```python
from build123d import *

# Parameters (mm, degrees)
SKETCH1_R           = 12.5
BOSS_EXTRUDE1_DEPTH = 115.4
SKETCH4_W           = 8
SKETCH4_H           = 8
CUT_EXTRUDE1_DEPTH  = 35.4
SKETCH11_R          = 15.5
BOSS_EXTRUDE4_DEPTH = 2
SKETCH12_R          = 12.5
SKETCH12_R_2        = 11.75
CUT_EXTRUDE2_DEPTH  = 1.2
SKETCH13_W          = 8
SKETCH13_H          = 7
CUT_EXTRUDE3_DEPTH  = 47
SKETCH16_R          = 12.5
SKETCH16_R_2        = 11.75
CUT_EXTRUDE5_DEPTH  = 1.2


with BuildPart() as part:
    # Sketch1 → Boss-Extrude1 (new body)
    with BuildSketch(Plane.XY):
        Circle(SKETCH1_R)
    extrude(amount=BOSS_EXTRUDE1_DEPTH)

    # Sketch4 → Cut-Extrude1 (cut)
    with BuildSketch(Plane(origin=(0, 0, 0), x_dir=(-1, 0, 0), z_dir=(0, 0, -1))):
        with Locations((0, 12.5)):
            Rectangle(SKETCH4_W, SKETCH4_H)
    extrude(amount=-CUT_EXTRUDE1_DEPTH, mode=Mode.SUBTRACT)

    # Sketch11 → Boss-Extrude4 (add)
    with BuildSketch(Plane(origin=(0, 0, 37.4), x_dir=(-1, 0, 0), z_dir=(0, 0, -1))):
        Circle(SKETCH11_R)
    extrude(amount=-BOSS_EXTRUDE4_DEPTH)

    # Sketch12 → Cut-Extrude2 (cut)
    with BuildSketch(Plane.XY.offset(60)):
        Circle(SKETCH12_R)
        Circle(SKETCH12_R_2, mode=Mode.SUBTRACT)
    extrude(amount=CUT_EXTRUDE2_DEPTH, mode=Mode.SUBTRACT)

    # Sketch13 → Cut-Extrude3 (cut)
    with BuildSketch(Plane.XY.offset(115.4)):
        with Locations((0, 12.5)):
            Rectangle(SKETCH13_W, SKETCH13_H)
    extrude(amount=-CUT_EXTRUDE3_DEPTH, mode=Mode.SUBTRACT)

    # Sketch16 → Cut-Extrude5 (cut)
    with BuildSketch(Plane.XY.offset(110.4)):
        Circle(SKETCH16_R)
        Circle(SKETCH16_R_2, mode=Mode.SUBTRACT)
    extrude(amount=CUT_EXTRUDE5_DEPTH, mode=Mode.SUBTRACT)


solid = part.part
```
For this review, take the finished solid that the model builds, in its own axes (mm). A direction names the side the tool comes from. Coordinates: 2 decimals unless noted, no trailing zeros. Order: outer loops, then holes, each group sorted by start corner. A loop starts at its lowest first (then second) coordinate and runs counter-clockwise, first axis right, second up. Notation, with made-up numbers: (61, -12) - (79, -12) arc R8 cw to (79, -1) - close; hole circle Ø11 at (9, -4.5). An arc over 180 degrees is marked (long way). Answer as a JSON object with one key per item and string values. Group by question number.
1. For faces 1 (the flat face through (0, 11, 68.4)), 2 (the flat face through (-4, 10, 17)), 3 (the cylindrical face through (11.923, 3.755, 49.556)), 4 (the cylindrical face through (-0.46, -11.74, 110.99)), list the 3-axis set-ups (+Z, -Z, +X, -X, +Y, -Y) from which the entire face can be reached by the end or side of a thin tool; tool diameter is ignored.
2. We need section D-D on z = 73. State the section outline as (x, y) points, then the cut area to 3 significant figures.
3. We need section C-C on z = 28.5. State the section outline as (x, y) points.
4. The part is to be moulded in two halves that separate along X. For faces 5 (the cylindrical face through (-2.71, -12.203, 18.438)), 6 (the flat face through (-4, 10, 92)), 7 (the flat face through (4, 10, 17)), 8 (the flat face through (0, 0, 115.4)), say which applies: pulls with the +X half, pulls with the -X half, needs draft (parallel to the pull), parting line crosses it, or undercut.
5. For probe 1 along X at (y, z) = (0, 35.5); probe 2 along Z at (x, y) = (-10, 10); probe 3 along X at (y, z) = (-11, 53), list the stretches that pass through material, from the lowest coordinate up.
6. We need section A-A on x = 0. State the section outline as (y, z) points, then the cut area to 3 significant figures.
7. We need section B-B on y = -5. State the section outline as (x, z) points.
8. Clearance check with flat-ended pins moving along their axes: P1, Ø1.5, axis at x = -10, y = -12, coming from the -Z side; P2, Ø9, axis at x = 1.5, z = 24.5, coming from the +Y side; P3, Ø3, axis at y = 4.5, z = 54, coming from the +X side. State where each tip first meets the part, or that it passes through.
Final values:
{
 "1": {"face 1": "+Z, +Y", "face 2": "-Z, +Y", "face 3": "+Z", "face 4": "none"},
 "2": {"outline": "(-4, 9) - (-4, 11.84) arc R12.5 ccw (long way) to (4, 11.84) - (4, 9) - close", "area": "465 mm²"},
 "3": {"outline": "(-4, 8.5) - (-4, 11.84) arc R12.5 ccw (long way) to (4, 11.84) - (4, 8.5) - close"},
 "4": {"face 5": "parting line crosses it", "face 6": "undercut", "face 7": "undercut", "face 8": "needs draft"},
 "5": {"probe 1": "-12.5 to 12.5", "probe 2": "37.4 to 39.4", "probe 3": "-5.94 to 5.94"},
 "6": {"outline": "(-15.5, 37.4) - (-12.5, 37.4) - (-12.5, 0) - (8.5, 0) - (8.5, 35.4) - (12.5, 35.4) - (12.5, 37.4) - (15.5, 37.4) - (15.5, 39.4) - (12.5, 39.4) - (12.5, 60) - (11.75, 60) - (11.75, 61.2) - (12.5, 61.2) - (12.5, 68.4) - (9, 68.4) - (9, 115.4) - (-12.5, 115.4) - (-12.5, 111.6) - (-11.75, 111.6) - (-11.75, 110.4) - (-12.5, 110.4) - (-12.5, 61.2) - (-11.75, 61.2) - (-11.75, 60) - (-12.5, 60) - (-12.5, 39.4) - (-15.5, 39.4) - close", "area": "2,590 mm²"},
 "7": {"outline": "(-14.67, 37.4) - (-11.46, 37.4) - (-11.46, 0) - (11.46, 0) - (11.46, 37.4) - (14.67, 37.4) - (14.67, 39.4) - (11.46, 39.4) - (11.46, 60) - (10.63, 60) - (10.63, 61.2) - (11.46, 61.2) - (11.46, 110.4) - (10.63, 110.4) - (10.63, 111.6) - (11.46, 111.6) - (11.46, 115.4) - (-11.46, 115.4) - (-11.46, 111.6) - (-10.63, 111.6) - (-10.63, 110.4) - (-11.46, 110.4) - (-11.46, 61.2) - (-10.63, 61.2) - (-10.63, 60) - (-11.46, 60) - (-11.46, 39.4) - (-14.67, 39.4) - close"},
 "8": {"P1": "z = 37.4", "P2": "y = 11.84", "P3": "x = 12.13"}
}
